```python
from build123d import *

# Parameters (mm, degrees)
SKETCH1_W           = 76.2
SKETCH1_H           = 50.8
BOSS_EXTRUDE1_DEPTH = 2.54
SKETCH2_W           = 50.8
SKETCH2_H           = 76.2
BOSS_EXTRUDE2_DEPTH = 8.89
CUT_EXTRUDE1_DEPTH  = 10.16
SKETCH4_W           = 8.89
SKETCH4_H           = 13.97
CUT_EXTRUDE2_DEPTH  = 48.195496607
SKETCH5_R           = 2.38125
CUT_EXTRUDE3_DEPTH  = 48.195496607
SKETCH9_W           = 23.749
SKETCH9_H           = 3.175
BOSS_EXTRUDE4_DEPTH = 7.62
FILLET1_R           = 1.5875
CHAMFER2_SIZE       = 0.79375


with BuildPart() as part:
    # Sketch1 → Boss-Extrude1 (new body)
    with BuildSketch(Plane(origin=(0, 0, 0), x_dir=(0, 1, 0), z_dir=(0, 0, 1))):
        Rectangle(SKETCH1_W, SKETCH1_H)
    extrude(amount=-BOSS_EXTRUDE1_DEPTH)

    # Sketch2 → Boss-Extrude2 (add)
    with BuildSketch(Plane.XY):
        Rectangle(SKETCH2_W, SKETCH2_H)
    extrude(amount=BOSS_EXTRUDE2_DEPTH)

    # Sketch3 → Cut-Extrude1 (cut)
    with BuildSketch(Plane.XY.offset(8.89)):
        Polygon((5.715, 19.05), (5.715, -19.05), (15.875, -19.05), (15.875, -6.985), (25.4, -6.985), (25.4, 6.985), (15.875, 6.985), (15.875, 19.05), align=None)
    extrude(amount=-CUT_EXTRUDE1_DEPTH, mode=Mode.SUBTRACT)

    # Sketch4 → Cut-Extrude2 (cut, through all)
    with BuildSketch(Plane.XY.offset(8.89)):
        with Locations((-20.955, 0)):
            Rectangle(SKETCH4_W, SKETCH4_H)
    extrude(amount=-CUT_EXTRUDE2_DEPTH, mode=Mode.SUBTRACT)

    # Sketch5 → Cut-Extrude3 (cut, through all)
    with BuildSketch(Plane.XY.offset(8.89)):
        with Locations((-17.78, -28.575)):
            Circle(SKETCH5_R)
        with Locations((-17.78, 28.575)):
            Circle(SKETCH5_R)
    extrude(amount=-CUT_EXTRUDE3_DEPTH, mode=Mode.SUBTRACT)

    # Sketch9 → Boss-Extrude4 (add)
    with BuildSketch(Plane.XY.offset(8.89)):
        with Locations((0, 28.575)):
            Rectangle(SKETCH9_W, SKETCH9_H)
        with Locations((0, -28.575)):
            Rectangle(SKETCH9_W, SKETCH9_H)
    extrude(amount=BOSS_EXTRUDE4_DEPTH)

    # Fillet1
    fillet1_edges = [part.edges().sort_by_distance(p)[0] for p in [
        (5.715, 19.05, 3.81),
        (15.875, 19.05, 3.81),
        (5.715, -19.05, 3.81),
        (15.875, -19.05, 3.81),
        (-16.51, 6.985, 3.175),
        (-16.51, -6.985, 3.175),
        (-11.8745, 30.1625, 12.7),
        (-11.8745, 26.9875, 12.7),
        (11.8745, 30.1625, 12.7),
        (11.8745, 26.9875, 12.7),
        (-11.8745, -26.9875, 12.7),
        (-11.8745, -30.1625, 12.7),
        (11.8745, -26.9875, 12.7),
        (11.8745, -30.1625, 12.7),
    ]]
    fillet(fillet1_edges, radius=FILLET1_R - 0.0001)  # a hair under: the kernel refuses the full size

    # Chamfer2
    chamfer2_edges = [part.edges().sort_by_distance(p)[0] for p in [
        (0, -26.9875, 16.51),
        (0, -30.1625, 16.51),
        (11.409561304, -29.697561304, 16.51),
        (11.409561304, -27.452438696, 16.51),
        (-11.409561304, -29.697561304, 16.51),
        (-11.409561304, -27.452438696, 16.51),
        (0, 30.1625, 16.51),
        (0, 26.9875, 16.51),
        (11.409561304, 27.452438696, 16.51),
        (11.409561304, 29.697561304, 16.51),
        (-11.409561304, 27.452438696, 16.51),
        (-11.409561304, 29.697561304, 16.51),
        (5.715, 0, 8.89),
        (10.795, 19.05, 8.89),
        (10.795, -19.05, 8.89),
        (15.875, -12.2238, 8.89),
        (6.179938696, 18.585061304, 8.89),
        (15.410061304, 18.585061304, 8.89),
        (6.179938696, -18.585061304, 8.89),
        (15.410061304, -18.585061304, 8.89),
        (20.6375, -6.985, 8.89),
        (20.6375, 6.985, 8.89),
        (15.875, 12.2238, 8.89),
    ]]
    chamfer(chamfer2_edges, length=CHAMFER2_SIZE)


solid = part.part
```
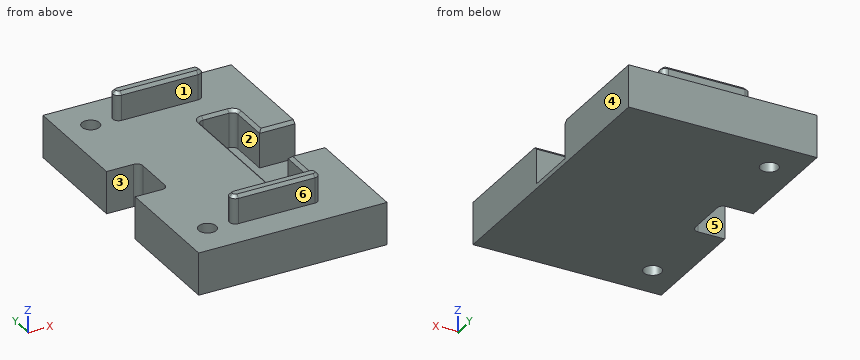
Design review of the part built by this model. Coordinates are the model's own, in mm. Face numbers are marked on the shaded views. A direction names the side the tool comes from. Coordinates: 2 decimals unless noted, no trailing zeros. Order: outer loops, then holes, each group sorted by start corner. A loop starts at its lowest first (then second) coordinate and runs counter-clockwise, first axis right, second up. Notation, with made-up numbers: M 73.5,56 L 111.5,56 A24 ccw 111.5,89 Z; hole C -17.5,41 d9. An arc over 180 degrees is marked long. Answer as a JSON object with one key per item and string values. Group by question number.
1) Mouldability with a two-part tool opening along Y and no side actions: class the marked faces 4, 5 and 6 as pulls with the +Y half, pulls with the -Y half, needs draft (parallel to the pull), parting line crosses it, or undercut.
2) Add section D-D, the plane z = 5.25. Count the separate pieces of the cut face and the enclosed holes in it, then the cut area to 3 significant figures.
3) For pin 1 (5 mm diameter, centred on x = -0.5, z = 12.5, fed in from +Y); pin 2 (15.5 mm diameter, centred on x = 12, y = 7.5, fed in from +Z); pin 3 (3 mm diameter, centred on y = -1, z = 2.5, fed in from -X); pin 4 (7.5 mm diameter, centred on x = 0, z = 11, fed in from +Y), all flat-tipped, find the tip position at first contact; note any pin that passes through.
4) Tool access review of the marked faces 1, 2 and 3: name each direction out of +Z, -Z, +X, -X, +Y, -Y from which nothing blocks a thin tool from reaching the whole face with its end or side.
5) Add section B-B, the plane y = -12. Write out the cut boundary in (x, z) (3 decimals), then the cut area to 3 significant figures.
6) Wall thickness on L1, parallel to X at y = -8, z = 0.25 (3 decimals); L2, parallel to Y at x = -0.5, z = 15; L3, parallel to Y at x = 10.5, z = 2.5: over which ranges is each line inside the solid? List them lowest first.
7) Add section C-C, the plane x = -2. Write out the cut boundary in (y, z), then the cut area to 3 significant figures.
Computed values:
{
 "1": {"face 4": "needs draft", "face 5": "undercut", "face 6": "pulls with the -Y half"},
 "2": {"separate pieces": "1", "enclosed holes": "2", "area": "3,190 mm^2"},
 "3": {"pin 1": "stops at y = 30.16", "pin 2": "stops at z = 8.89", "pin 3": "stops at x = -16.51", "pin 4": "stops at y = 38.1"},
 "4": {"face 1": "+Z, +X, -X", "face 2": "+Z", "face 3": "+Z, -Z, -X"},
 "5": {"outline": "M -25.4,-2.54 L 25.4,-2.54 L 25.4,8.89 L 16.669,8.89 L 15.875,8.096 L 15.875,-1.27 L 5.715,-1.27 L 5.715,8.096 L 4.921,8.89 L -25.4,8.89 Z", "area": "477 mm^2"},
 "6": {"L1": "x = -25.4 to 5.715, 15.875 to 25.4", "L2": "y = -30.16 to -26.99, 26.99 to 30.16", "L3": "y = -38.1 to -19.05, 19.05 to 38.1"},
 "7": {"outline": "M -38.1,-2.54 L 38.1,-2.54 L 38.1,8.89 L 30.16,8.89 L 30.16,15.72 L 29.37,16.51 L 27.78,16.51 L 26.99,15.72 L 26.99,8.89 L -26.99,8.89 L -26.99,15.72 L -27.78,16.51 L -29.37,16.51 L -30.16,15.72 L -30.16,8.89 L -38.1,8.89 Z", "area": "918 mm^2"}
}
